For this review, take the finished solid that the model builds, in its own axes (mm). Round coordinates to 2 decimals unless told otherwise and drop trailing zeros. Loops run counter-clockwise (first coordinate to the right, second up) from the corner with the lowest first, then second, coordinate; pieces in that order, holes last. Notation, with made-up numbers: (63, 68) -> (113, 68) arc R24 ccw to (113, 78) -> close; hole circle Ø7 at (83.5, -22.5). An arc over 180 degrees is marked (long way). Write each question's results on one line, items separated by ' | '.
```python
from build123d import *

# Parameters (mm, degrees)
BOSS_EXTRUDE1_DEPTH        = 30.2895
F_10_32_TAPPED_HOLE1_D     = 4.0386
F_10_32_TAPPED_HOLE1_DEPTH = 12.02944
F_10_32_TAPPED_HOLE1_TIP   = 1.213317848
F_10_32_TAPPED_HOLE2_D     = 4.0386
F_10_32_TAPPED_HOLE2_DEPTH = 12.02944
F_10_32_TAPPED_HOLE2_TIP   = 1.213317848


with BuildPart() as part:
    # Sketch1 → Boss-Extrude1 (new, symmetric)
    with BuildSketch(Plane.XY):
        with BuildLine():
            ThreePointArc((6.35, 2.48767683), (5.906206651, 3.40995), (5.329391331, 4.255422899))
            Line((5.329391331, 4.255422899), (1.020608669, 6.743099729))
            ThreePointArc((1.020608669, 6.743099729), (0, 6.8199), (-1.020608669, 6.743099729))
            Line((-1.020608669, 6.743099729), (-5.329391331, 4.255422899))
            ThreePointArc((-5.329391331, 4.255422899), (-5.906206651, 3.40995), (-6.35, 2.48767683))
            Line((-6.35, 2.48767683), (-6.35, -2.48767683))
            ThreePointArc((-6.35, -2.48767683), (-5.906206651, -3.40995), (-5.329391331, -4.255422899))
            Line((-5.329391331, -4.255422899), (-1.020608669, -6.743099729))
            ThreePointArc((-1.020608669, -6.743099729), (0, -6.8199), (1.020608669, -6.743099729))
            Line((1.020608669, -6.743099729), (5.329391331, -4.255422899))
            ThreePointArc((5.329391331, -4.255422899), (5.906206651, -3.40995), (6.35, -2.48767683))
            Line((6.35, -2.48767683), (6.35, 2.48767683))
        make_face()
    extrude(amount=BOSS_EXTRUDE1_DEPTH, both=True)

    # #10-32 Tapped Hole1
    with Locations(Plane.XY.offset(30.2895)):
        with Locations((0, 0)):
            Hole(F_10_32_TAPPED_HOLE1_D / 2, depth=F_10_32_TAPPED_HOLE1_DEPTH)
            with Locations((0, 0, -(F_10_32_TAPPED_HOLE1_DEPTH + F_10_32_TAPPED_HOLE1_TIP / 2))):  # 118° drill point
                Cone(0, F_10_32_TAPPED_HOLE1_D / 2, F_10_32_TAPPED_HOLE1_TIP, mode=Mode.SUBTRACT)

    # #10-32 Tapped Hole2
    with Locations(Plane(origin=(0, 0, -30.2895), x_dir=(-1, 0, 0), z_dir=(0, 0, -1))):
        with Locations((0, 0)):
            Hole(F_10_32_TAPPED_HOLE2_D / 2, depth=F_10_32_TAPPED_HOLE2_DEPTH)
            with Locations((0, 0, -(F_10_32_TAPPED_HOLE2_DEPTH + F_10_32_TAPPED_HOLE2_TIP / 2))):  # 118° drill point
                Cone(0, F_10_32_TAPPED_HOLE2_D / 2, F_10_32_TAPPED_HOLE2_TIP, mode=Mode.SUBTRACT)


solid = part.part
```
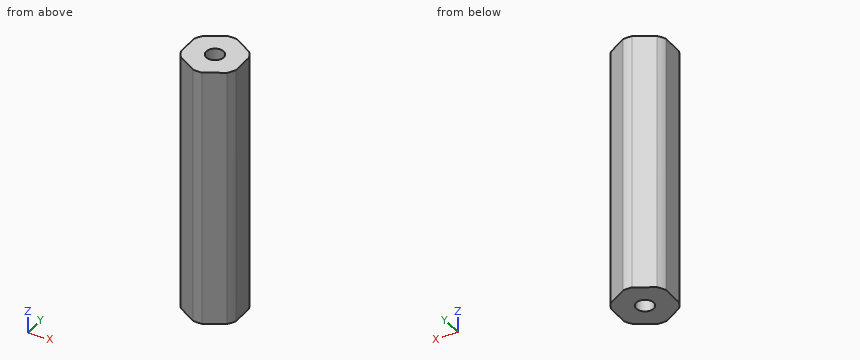
1. Consider section A-A (z = 10). State the section outline as (x, y) points, plus the area to 3 significant figures.
Values found:
outline: (-6.35, -2.49) arc R6.82 ccw to (-5.33, -4.26) -> (-1.02, -6.74) arc R6.82 ccw to (1.02, -6.74) -> (5.33, -4.26) arc R6.82 ccw to (6.35, -2.49) -> (6.35, 2.49) arc R6.82 ccw to (5.33, 4.26) -> (1.02, 6.74) arc R6.82 ccw to (-1.02, 6.74) -> (-5.33, 4.26) arc R6.82 ccw to (-6.35, 2.49) -> close | area: 137 mm2
2. To check wall thickness, follow probe 1 along Y at (x, z) = (0, 26.75); probe 2 along X at (y, z) = (0, -22.5); probe 3 along X at (y, z) = (2.5, -10). State the ranges of each line that lie inside material, in increasing order.
Values found:
probe 1: y = -6.82 to -2.02, 2.02 to 6.82 | probe 2: x = -6.35 to -2.02, 2.02 to 6.35 | probe 3: x = -6.35 to 6.35
3. Consider section B-B (x = 4.25). State the section outline as (y, z) points.
Values found:
outline: (-4.88, -30.29) -> (4.88, -30.29) -> (4.88, 30.29) -> (-4.88, 30.29) -> close
4. For pin 1 (1 mm diameter, centred on x = 3, z = -5.5, fed in from +Y); pin 2 (2.5 mm diameter, centred on x = 0, y = 0, fed in from -Z); pin 3 (5 mm diameter, centred on x = 3, z = 17, fed in from -Y), all flat-tipped, find the tip position at first contact; note any pin that passes through.
Values found:
pin 1: stops at y = 5.89 | pin 2: stops at z = -17.8 | pin 3: stops at y = -6.8
